from build123d import *

# Parameters (mm, degrees)
SKETCH1_R           = 3
BOSS_EXTRUDE1_DEPTH = 22.7
SKETCH3_R           = 0.2
SKETCH5_R           = 0.2


with BuildPart() as part:
    # Sketch1 → Boss-Extrude1 (new body)
    with BuildSketch(Plane(origin=(0, 0, 0), x_dir=(1, 0, 0), z_dir=(0, 1, 0))):
        with Locations(Location((0, 0, 0), (0, 0, 270))):
            Circle(SKETCH1_R)
    extrude(amount=BOSS_EXTRUDE1_DEPTH)

    # Sweep1: sweep along a path in Sketch2
    with BuildLine(Plane.XY) as sweep1_path:
        Line((2.8, 22.7), (2.8, 38.7))
        ThreePointArc((2.8, 38.7), (-0.2, 41.7), (-3.2, 38.7))
    # Sketch3 → Sweep1 (sweep)
    with BuildSketch(Plane(origin=(0, 22.7, 0), x_dir=(1, 0, 0), z_dir=(0, 1, 0))):
        with Locations((2.8, 0)):
            Circle(SKETCH3_R)
    sweep(path=sweep1_path.line)

    # Sweep2: sweep along a path in Sketch4
    with BuildLine(Plane.XY) as sweep2_path:
        Line((-2.8, 0), (-2.8, -6))
        ThreePointArc((-2.8, -6), (0.2, -9), (3.2, -6))
    # Sketch5 → Sweep2 (sweep)
    with BuildSketch(Plane.XZ):
        with Locations((-2.8, 0)):
            Circle(SKETCH5_R)
    sweep(path=sweep2_path.line)


solid = part.part
Part model, mm, in its own coordinate system. Round coordinates to 2 decimals unless told otherwise and drop trailing zeros. Write each loop counter-clockwise with the first axis right and the second up, starting at its lowest first coordinate (ties: lowest second). Pieces come first, ordered by that corner, then holes. Notation, with made-up numbers: M 0.5,-34.75 L 38.5,-34.75 A23 ccw 38.5,-9.75 Z; hole C 17.5,-4.75 d8. An arc over 180 degrees is marked long. Return JSON: item names as keys, results as strings. Group by question number.
(1) Saw through at C-C on y = 20. Write the cut outline in (x, z).
(2) Saw through at A-A on y = 26.5. Write the cut outline in (x, z), then the cut area to 3 significant figures.
(3) Pin check, flat tips, straight feed: pin 1 Ø1 at (x, z) = (2, -1) entering from +Y; pin 2 Ø3 at (x, z) = (-0.5, 0.5) entering from +Y; pin 3 Ø2 at (x, z) = (-1, -2) entering from -Y; pin 4 Ø4 at (x, y) = (2.5, 2) entering from +Z. Stop position of each tip, or through.
(4) Drill centre lines: probe 1 along Y at (x, z) = (0, 1.5); probe 2 along X at (y, z) = (3, -0.05); probe 3 along Z at (x, y) = (-0.25, 20). Where is each one in solid material? Low to high.
(5) Saw through at B-B on x = 0. Count the separate pieces of the cut face and the enclosed holes in it, then the cut area to 3 significant figures.
Returned:
{
 "1": {"outline": "C 0,0 d6"},
 "2": {"outline": "C 2.8,0 d0.4", "area": "0.126 mm²"},
 "3": {"pin 1": "y = 22.7", "pin 2": "y = 41.9", "pin 3": "y = 0", "pin 4": "z = 2.96"},
 "4": {"probe 1": "0 to 22.7", "probe 2": "-3 to 3", "probe 3": "-2.99 to 2.99"},
 "5": {"separate pieces": "3", "enclosed holes": "0", "area": "136 mm²"}
}
